Autodesk Inventor part; units mm, degrees
ref_plane "YZ Plane" through (0, 0, 0) normal (1, 0, 0) x (0, 1, 0)
ref_plane "XZ Plane" through (0, 0, 0) normal (0, 1, 0) x (-1, 0, 0)
ref_plane "XY Plane" through (0, 0, 0) normal (0, 0, 1) x (1, 0, 0)
sketch "Sketch1" plane through (0, 0, 0) normal (0, 0, 1) x (1, 0, 0)
  line L0 (0, 0) -> (148, 0)
  line L1 (148, 0) -> (148, 210)
  line L2 (148, 210) -> (0, 210)
  line L3 (0, 210) -> (0, 0)
  dimension "d0" = 148
  dimension "d1" = 210
extrude "Extrusion1" add sketch "Sketch1" along normal blind 3
sketch "Sketch2" plane through (0, 0, 3) normal (0, 0, 1) x (1, 0, 0)
  line L0 (0, 0) -> (0, 210)
  line L1 (148, 0) -> (0, 0)
  line L2 (148, 210) -> (148, 0)
  line L3 (0, 210) -> (148, 210)
  line L4 (4, 185) -> (7, 185)
  line L5 (7, 185) -> (7, 175)
  line L6 (7, 175) -> (4, 175)
  line L7 (4, 175) -> (4, 185)
  line L8 (4, 40) -> (7, 40)
  line L9 (7, 40) -> (7, 30)
  line L10 (7, 30) -> (4, 30)
  line L11 (4, 30) -> (4, 40)
  line L12 (4, 20) -> (7, 20)
  line L13 (7, 20) -> (7, 10)
  line L14 (7, 10) -> (4, 10)
  line L15 (4, 10) -> (4, 20)
  line L16 (141, 175) -> (144, 175)
  line L17 (144, 175) -> (144, 185)
  line L18 (144, 185) -> (141, 185)
  line L19 (141, 185) -> (141, 175)
  line L20 (141, 40) -> (144, 40)
  line L21 (144, 40) -> (144, 30)
  line L22 (144, 30) -> (141, 30)
  line L23 (141, 30) -> (141, 40)
  line L24 (141, 20) -> (144, 20)
  line L25 (144, 20) -> (144, 10)
  line L26 (144, 10) -> (141, 10)
  line L27 (141, 10) -> (141, 20)
  dimension "d4" = 4
  dimension "d5" = 3
  dimension "d6" = 10
  dimension "d7" = 25
  dimension "d10" = 10
  dimension "d11" = 10
  dimension "d12" = 10
  dimension "d13" = 10
  dimension "d14" = 3
  dimension "d15" = 4
  dimension "d17" = 10
  dimension "d18" = 10
  dimension "d19" = 10
  dimension "d43" = 4
  dimension "d44" = 4
  dimension "d45" = 3
  dimension "d46" = 3
  dimension "d51" = 4
  dimension "d52" = 3
  dimension "d165" = 10
  dimension "d166" = 25
  dimension "d169" = 3
extrude "Extrusion2" cut sketch "Sketch2" against normal through all contours L4 L5 L6 L7 | L8 L9 L10 L11 | L12 L13 L14 L15 | L19 L18 L17 L16 | L20 L21 L22 L23 | L24 L25 L26 L27
sketch "Sketch3" plane through (0, 0, 3) normal (0, 0, 1) x (1, 0, 0)
  line L0 (7, 30) -> (4, 30)
  line L1 (0, 210) -> (148, 210)
  line L2 (4, 175) -> (4, 185)
  line L3 (141, 175) -> (141, 185)
  line L4 (7, 40) -> (7, 30)
  point P0 (5.5, 190)
  point P1 (142.5, 190)
  point P2 (5.5, 25)
  point P3 (142.5, 25)
  point P4 (141, 30)
  dimension "d24" = 5
  dimension "d54" = 1.5
  dimension "d162" = 20
  dimension "d163" = 20
  dimension "d167" = 1.5
  dimension "d168" = 1.5
  dimension "d170" = 1.5
hole "Hole1" at (5.5, 190, 3) at (142.5, 190, 3) at (5.5, 25, 3) at (142.5, 25, 3) direction (0, 0, -1) diameter 3 end through all
sketch "草圖12" plane through (0, 0, 3) normal (0, 0, 1) x (1, 0, 0)
  line L0 (0, 0) -> (0, 210)
  line L1 (148, 0) -> (0, 0)
  line L2 (148, 210) -> (148, 0)
  line L3 (0, 210) -> (148, 210)
  line L4 (32, 204.5) -> (42, 204.5)
  line L5 (42, 204.5) -> (42, 201.5)
  line L6 (42, 201.5) -> (32, 201.5)
  line L7 (32, 201.5) -> (32, 204.5)
  line L8 (106, 201.5) -> (116, 201.5)
  line L9 (116, 201.5) -> (116, 204.5)
  line L10 (116, 204.5) -> (106, 204.5)
  line L11 (106, 204.5) -> (106, 201.5)
  line L12 (32, 23.5) -> (42, 23.5)
  line L13 (42, 23.5) -> (42, 26.5)
  line L14 (42, 26.5) -> (32, 26.5)
  line L15 (32, 26.5) -> (32, 23.5)
  line L16 (106, 26.5) -> (116, 26.5)
  line L17 (116, 26.5) -> (116, 23.5)
  line L18 (116, 23.5) -> (106, 23.5)
  line L19 (106, 23.5) -> (106, 26.5)
  dimension "d148" = 3
  dimension "d150" = 10
  dimension "d151" = 32
  dimension "d152" = 5.5
  dimension "d153" = 10
  dimension "d154" = 32
  dimension "d155" = 3
  dimension "d156" = 23.5
  dimension "d157" = 32
  dimension "d158" = 32
extrude "擠出5" cut sketch "草圖12" against normal through all contours L4 L5 L6 L7 | L11 L10 L9 L8 | L15 L14 L13 L12 | L16 L17 L18 L19
fillet "圓角3" radius 2 4 edges at (0, 0, 1.5) (148, 0, 1.5) (0, 210, 1.5) (148, 210, 1.5)
properties part number "plastic_part_1"
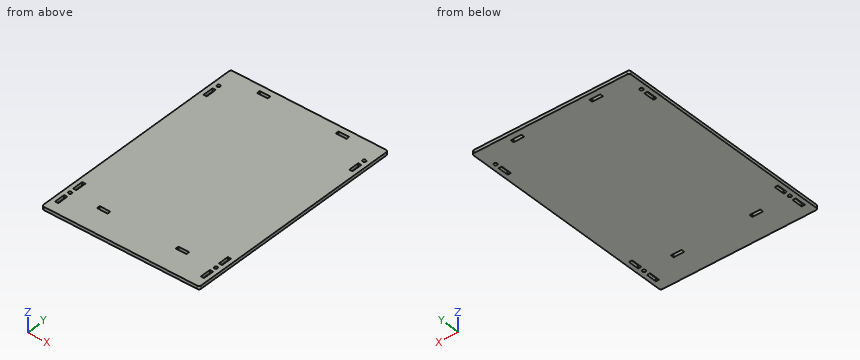
Build history of the part. All positions in model axes, mm. Give positions to 0.01 mm unless a question says otherwise; leave off trailing zeros. Loops run counter-clockwise (first coordinate to the right, second up) from the corner with the lowest first, then second, coordinate; pieces in that order, holes last. Notation, with made-up numbers: (70, 50) - (106, 50) arc R25 ccw to (106, 88) - close; hole circle Ø6 at (68.5, -35). An arc over 180 degrees is marked (long way). Use a Markdown table: item, result.
(1) Band-saw the part on A-A (x = 109.5). Give the cut face in (y, z), and give its area (3 significant figures).
Taken from the geometry:
| item | result |
|---|---|
| outline | (0, 0) - (23.5, 0) - (23.5, 3) - (0, 3) - close; (26.5, 0) - (201.5, 0) - (201.5, 3) - (26.5, 3) - close; (204.5, 0) - (210, 0) - (210, 3) - (204.5, 3) - close |
| area | 612 mm2 |
(2) Drop a flat-ended pin along its axis: pin 1 Ø1.5 at (x, z) = (39, 1.5) entering from -Y. Give the stop position or say it passes through.
Taken from the geometry:
| item | result |
|---|---|
| pin 1 | y = 0 |
(3) Wall check: line 1 along X through (y, z) = (190, 1.7); line 2 along X through (y, z) = (25, 2.2); line 3 along Y through (x, z) = (5.5, 1.4). Give the ranges that are in metal, low to high.
Taken from the geometry:
| item | result |
|---|---|
| line 1 | 0 to 4, 7 to 141, 144 to 148 |
| line 2 | 0 to 4, 7 to 32, 42 to 106, 116 to 141, 144 to 148 |
| line 3 | 0 to 10, 20 to 23.5, 26.5 to 30, 40 to 175, 185 to 188.5, 191.5 to 210 |
(4) Band-saw the part on B-B (y = 181). Give the cut face in (x, z), and give its area (3 significant figures).
Taken from the geometry:
| item | result |
|---|---|
| outline | (0, 0) - (4, 0) - (4, 3) - (0, 3) - close; (7, 0) - (141, 0) - (141, 3) - (7, 3) - close; (144, 0) - (148, 0) - (148, 3) - (144, 3) - close |
| area | 426 mm2 |
